```python
from build123d import *

# Parameters (mm, degrees)
SKETCH1_W           = 45
SKETCH1_H           = 34
BOSS_EXTRUDE1_DEPTH = 4
SKETCH2_W           = 45
SKETCH2_H           = 4
BOSS_EXTRUDE2_DEPTH = 20
SKETCH3_R           = 2
CUT_EXTRUDE1_DEPTH  = 10


with BuildPart() as part:
    # Sketch1 → Boss-Extrude1 (new body)
    with BuildSketch(Plane.XY):
        with Locations((22.5, 17)):
            Rectangle(SKETCH1_W, SKETCH1_H)
    extrude(amount=BOSS_EXTRUDE1_DEPTH)

    # Sketch2 → Boss-Extrude2 (add)
    with BuildSketch(Plane.XY.offset(4)):
        with Locations((22.5, 2)):
            Rectangle(SKETCH2_W, SKETCH2_H)
    extrude(amount=BOSS_EXTRUDE2_DEPTH)

    # Sketch3 → Cut-Extrude1 (cut)
    with BuildSketch(Plane.XY.offset(4)):
        with Locations((5, 18)):
            Circle(SKETCH3_R)
        with Locations((40, 18)):
            Circle(SKETCH3_R)
    extrude(amount=-CUT_EXTRUDE1_DEPTH, mode=Mode.SUBTRACT)


solid = part.part
```
Source: CAD feature listing. Evaluate the final solid. Frame: model axes, mm. A direction names the side the tool comes from. Give positions to 0.01 mm unless a question says otherwise; leave off trailing zeros. Loops run counter-clockwise (first coordinate to the right, second up) from the corner with the lowest first, then second, coordinate; pieces in that order, holes last. Notation, with made-up numbers: (-15, 85.25) - (2, 85.25) arc R17 ccw to (2, 103.25) - close; hole circle Ø3 at (11, 36.5). An arc over 180 degrees is marked (long way). Use CSV: the item, a comma, the result in double quotes. Start each with the question number.
1. Pin query (flat end, axial travel): pin 1 (8 mm diameter, centred on x = 34.5, y = 23.5, fed in from +Z); pin 2 (6 mm diameter, centred on x = 30, z = 16, fed in from -Y); pin 3 (2 mm diameter, centred on x = 6.5, z = 6.5, fed in from +Y). Return the tip coordinate at first contact, or that it passes through.
2. Section B-B (x = 5). Output: boundary loops of the cut face in (y, z), then the cut area to 3 significant figures.
3. Section A-A (y = 18). Output: boundary loops of the cut face in (x, z), then the cut area to 3 significant figures.
4. Section D-D (x = 13.5). Output: boundary loops of the cut face in (y, z), then the cut area to 3 significant figures.
5. Ray query, L1, parallel to Y at x = 5, z = 1.7; L2, parallel to Y at x = 2, z = 15.25. Return the intervals inside material, ascending.
6. Reachability of faces 4 (the flat face through (22, 34, 2)), 5 (the flat face through (22, 4, 14)) from +Z, -Z, +X, -X, +Y, -Y: full face, straight path, thin tool, end or side. Return the list, or none.
7. Section C-C (z = 13.75). Output: boundary loops of the cut face in (x, y), then the cut area to 3 significant figures.
8. Draft query along X for faces 1 (the cylindrical face through (5, 20, 2)), 2 (the flat face through (0, 12, 3)), 3 (the flat face through (22, 17, 0)). Return one class per face: +X half, -X half, draft (parallel to the pull), parting line (faces both ways), or undercut.
Response:
1,pin 1,"z = 4"
1,pin 2,"y = 0"
1,pin 3,"y = 4"
2,outline,"(0, 0) - (16, 0) - (16, 4) - (4, 4) - (4, 24) - (0, 24) - close; (20, 0) - (34, 0) - (34, 4) - (20, 4) - close"
2,area,"200 mm²"
3,outline,"(0, 0) - (3, 0) - (3, 4) - (0, 4) - close; (7, 0) - (38, 0) - (38, 4) - (7, 4) - close; (42, 0) - (45, 0) - (45, 4) - (42, 4) - close"
3,area,"148 mm²"
4,outline,"(0, 0) - (34, 0) - (34, 4) - (4, 4) - (4, 24) - (0, 24) - close"
4,area,"216 mm²"
5,L1,"0 to 16, 20 to 34"
5,L2,"0 to 4"
6,face 4,"+Z, -Z, +X, -X, +Y"
6,face 5,"+Z, +X, -X, +Y"
7,outline,"(0, 0) - (45, 0) - (45, 4) - (0, 4) - close"
7,area,"180 mm²"
8,face 1,"undercut"
8,face 2,"-X half"
8,face 3,"draft"
